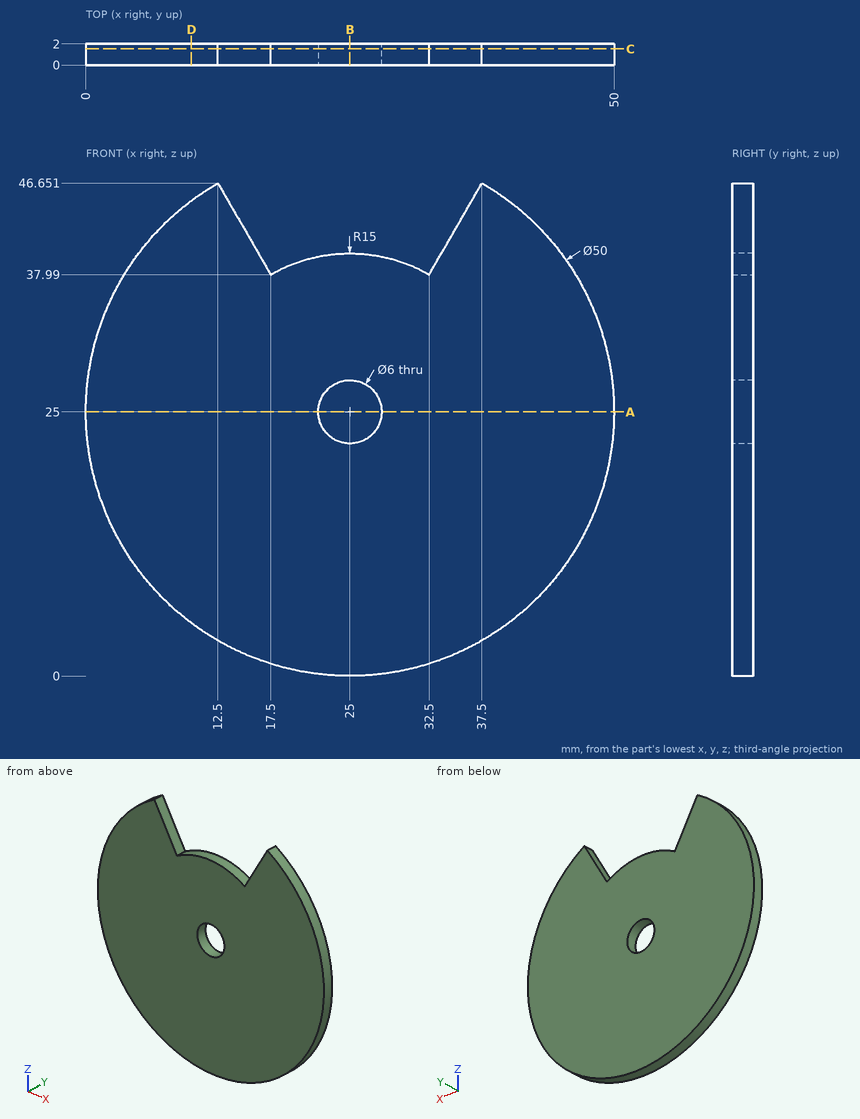
Geometry: see drawing. Coordinates: mm, zero at the bounding-box minimum. Round coordinates to 2 decimals unless told otherwise and drop trailing zeros. Loops run counter-clockwise (first coordinate to the right, second up) from the corner with the lowest first, then second, coordinate; pieces in that order, holes last. Notation, with made-up numbers: (11, 34) - (68, 34) arc R30 ccw to (68, 60) - close; hole circle Ø11 at (-35, 3). An arc over 180 degrees is marked (long way). One line per item, written item: value. Start each with the question number.
(1) Section C-C, the plane y = 1.55. Return loops of the section in (x, z).
(2) Section B-B, the plane x = 25. Return loops of the section in (y, z).
(3) Contact query for flat-ended pins moving along their axis: P1, Ø1, axis at y = 0.5, z = 37.5, coming from the +X side; P2, Ø1, axis at y = 1, z = 39, coming from the +X side; P3, Ø12, axis at x = 8, z = 20, coming from the -Y side. Output: stop coordinate, or through.
(4) Section D-D, the plane x = 10. Return loops of the section in (y, z).
(5) Section A-A, the plane z = 25. Return loops of the section in (x, y).
(6) Ray query, line 1 (Z direction, x = 25, y = 0.8); line 2 (Z direction, x = 24, y = 0.35); line 3 (X direction, y = 1.8, z = 44.5) (1 decimal). Return the intervals inside material, ascending. Write a range as [from, to].
Results below:
1. outline: (12.5, 46.65) arc R25 ccw (long way) to (37.5, 46.65) - (32.5, 37.99) arc R15 ccw to (17.5, 37.99) - close; hole circle Ø6 at (25, 25)
2. outline: (0, 0) - (2, 0) - (2, 22) - (0, 22) - close; (0, 28) - (2, 28) - (2, 40) - (0, 40) - close
3. P1: x = 46.93
3. P2: x = 46.04
3. P3: y = 0
4. outline: (0, 5) - (2, 5) - (2, 45) - (0, 45) - close
5. outline: (0, 0) - (22, 0) - (22, 2) - (0, 2) - close; (28, 0) - (50, 0) - (50, 2) - (28, 2) - close
6. line 1: [0, 22], [28, 40]
6. line 2: [0.02, 22.17], [27.83, 39.97]
6. line 3: [9.4, 13.7], [36.3, 40.6]
